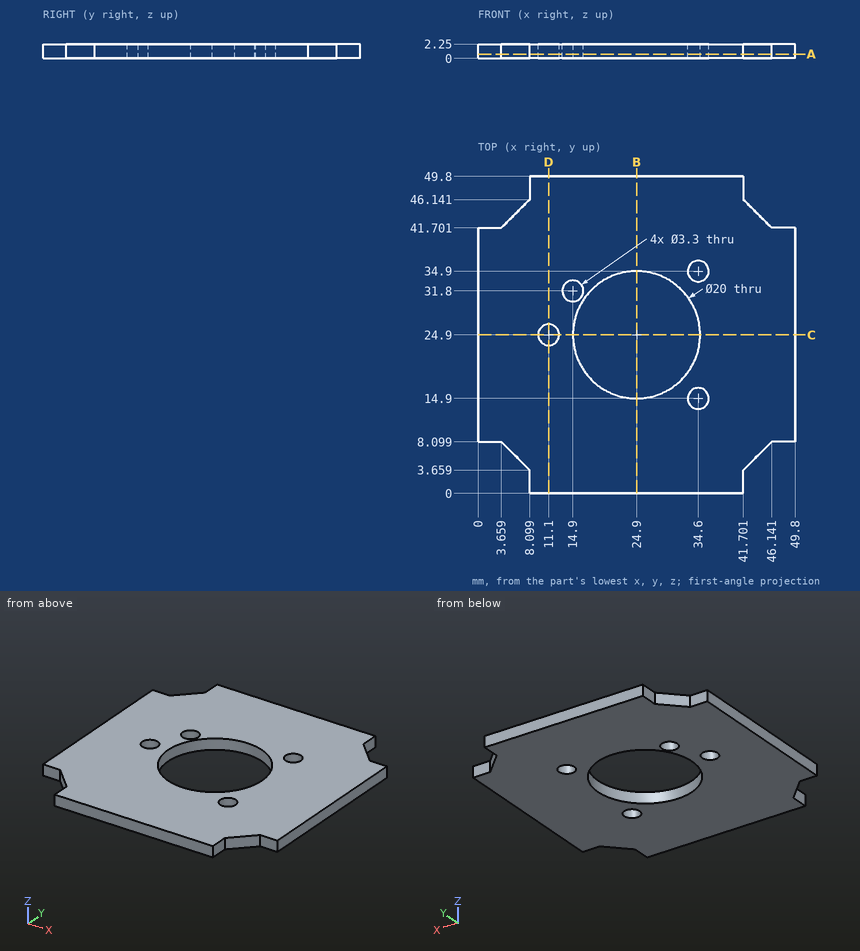
Answer from the drawing. Dimensions are ordinates in mm from the lowest x, y and z of the part. Round coordinates to 2 decimals unless told otherwise and drop trailing zeros. Order: outer loops, then holes, each group sorted by start corner. A loop starts at its lowest first (then second) coordinate and runs counter-clockwise, first axis right, second up.
1) The part is cut by section A-A on z = 0.65. Write down the section's boundary in (x, y), plus the area to 3 significant figures.
2) The part is cut by section B-B on x = 24.9. Write down the section's boundary in (y, z).
3) The part is cut by section C-C on y = 24.9. Write down the section's boundary in (x, z).
4) Straight lines are drawn through the part: L1, parallel to Y at x = 11.1, z = 0.95; L2, parallel to Y at x = 24.9, z = 1.7; L3, parallel to X at y = 26, z = 1.05. For each, find the intervals that lie inside material, in ascending order.
5) Flat-ended cylindrical pins translate along their axes: pin 1 (1.1 mm diameter, centred on x = 2, z = 1.5, fed in from -Y); pin 2 (1.1 mm diameter, centred on x = 48.5, z = 1, fed in from +Y); pin 3 (1.1 mm diameter, centred on y = 48, z = 1, fed in from -X). Find the tip coordinate at first contact, or state that the pin passes through.
6) The part is cut by section D-D on x = 11.1. Write down the section's boundary in (y, z).
Resolved:
1. outline: (0, 8.1) - (3.66, 8.1) - (8.1, 3.66) - (8.1, 0) - (41.7, 0) - (41.7, 3.66) - (46.14, 8.1) - (49.8, 8.1) - (49.8, 41.7) - (46.14, 41.7) - (41.7, 46.14) - (41.7, 49.8) - (8.1, 49.8) - (8.1, 46.14) - (3.66, 41.7) - (0, 41.7) - close; hole circle Ø3.3 at (11.1, 24.9); hole circle Ø3.3 at (14.9, 31.8); hole circle Ø20 at (24.9, 24.9); hole circle Ø3.3 at (34.6, 14.9); hole circle Ø3.3 at (34.6, 34.9)
1. area: 1,910 mm2
2. outline: (0, 0) - (14.9, 0) - (14.9, 2.25) - (0, 2.25) - close; (34.9, 0) - (49.8, 0) - (49.8, 2.25) - (34.9, 2.25) - close
3. outline: (0, 0) - (9.45, 0) - (9.45, 2.25) - (0, 2.25) - close; (12.75, 0) - (14.9, 0) - (14.9, 2.25) - (12.75, 2.25) - close; (34.9, 0) - (49.8, 0) - (49.8, 2.25) - (34.9, 2.25) - close
4. L1: y = 0 to 23.25, 26.55 to 49.8
4. L2: y = 0 to 14.9, 34.9 to 49.8
4. L3: x = 0 to 9.87, 12.33 to 14.96, 34.84 to 49.8
5. pin 1: stops at y = 8.1
5. pin 2: stops at y = 41.7
5. pin 3: stops at x = 8.1
6. outline: (0, 0) - (23.25, 0) - (23.25, 2.25) - (0, 2.25) - close; (26.55, 0) - (49.8, 0) - (49.8, 2.25) - (26.55, 2.25) - close
